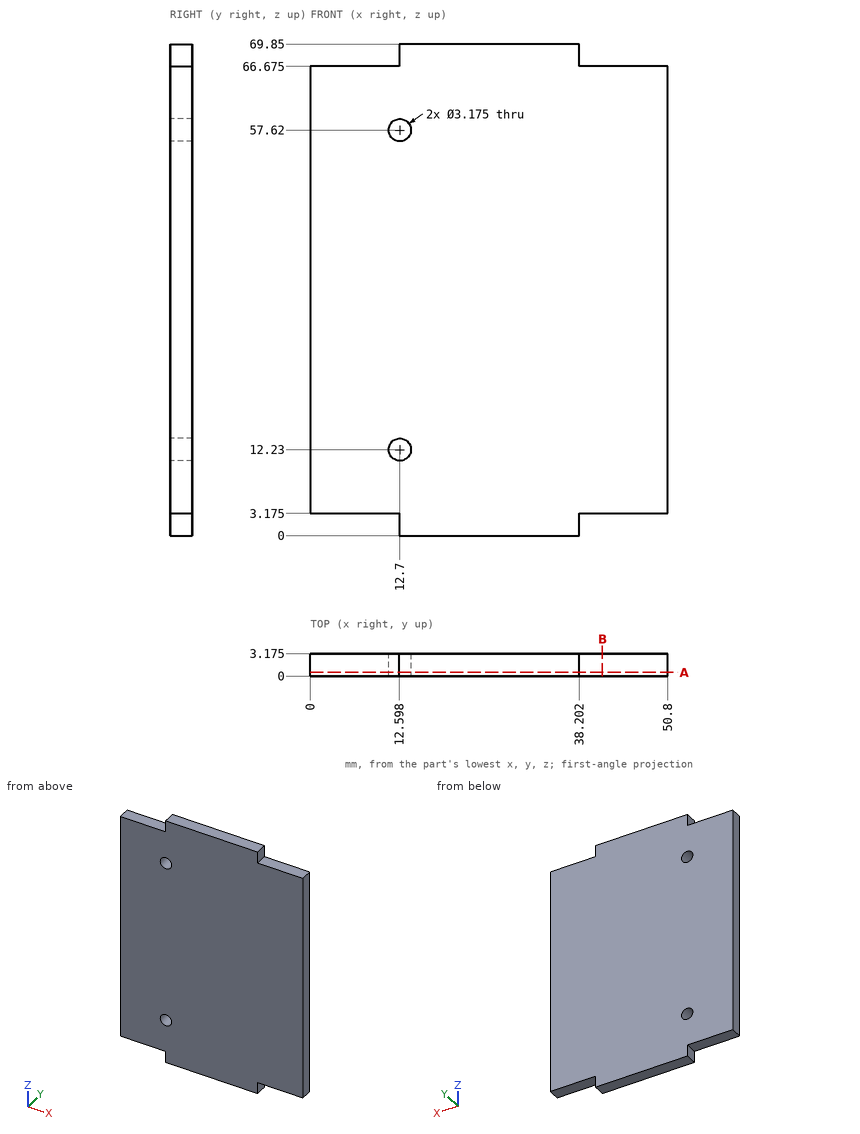
Geometry check sheet. Reference: drawing and pictorial views, mm from the part's lowest x, y, z. Round coordinates to 2 decimals unless told otherwise and drop trailing zeros. Loops run counter-clockwise (first coordinate to the right, second up) from the corner with the lowest first, then second, coordinate; pieces in that order, holes last. Notation, with made-up numbers: (75, -12.5) - (111, -12.5) arc R22 ccw to (111, -3.5) - close; hole circle Ø6 at (-37.75, 87). An arc over 180 degrees is marked (long way). Write item = value, one per line. Start each with the question number.
Q1. Thickness scan on L1, parallel to Z at x = 12.7, y = 1.7; L2, parallel to Z at x = 43.5, y = 2.5 (1 decimal). Record the ranges inside material, lowest first.
Q2. Section check A-A (y = 0.5). Count the separate pieces of the cut face and the enclosed holes in it, plus the area to 3 significant figures.
Q3. Depth check by flat-ended pin: P1, Ø3.5, axis at x = 12.7, z = 12.23, coming from the -Y side; P2, Ø1.9, axis at x = 12.7, z = 57.62, coming from the -Y side; P3, Ø1.6, axis at x = 8.5, y = 1, coming from the +Z side (3 decimals); P4, Ø1, axis at y = 2, z = 2, coming from the -X side. Enter the tip coordinate at first touch or a pass-through.
Q4. Section check B-B (x = 41.5). Record the boundary of the cut face in (y, z) (1 decimal), plus the area to 3 significant figures.
Derived:
q1.L1 = 0 to 10.64, 13.82 to 56.03, 59.21 to 69.85
q1.L2 = 3.2 to 66.7
q2.separate_pieces = 1
q2.enclosed_holes = 2
q2.area = 3,370 mm^2
q3.P1 = 0
q3.P2 = through
q3.P3 = 66.675
q3.P4 = 12.6
q4.outline = (0, 3.2) - (3.2, 3.2) - (3.2, 66.7) - (0, 66.7) - close
q4.area = 202 mm^2
